```python
from build123d import *

# Parameters (mm, degrees)
F0_W     = 126
F0_H     = 73
F1_DEPTH = 2
F2_W     = 1.7
F2_H     = 1.5
F2_W_2   = 19.1
F2_H_2   = 70
F3_DEPTH = 19
F5_DEPTH = 100
F6_R     = 0.1


with BuildPart() as f1:
    # F0 (on Top) → F1 (new body)
    with BuildSketch(Plane.XY):
        Rectangle(F0_W, F0_H)
    extrude(amount=F1_DEPTH)

    # F2 (on face) → F3 (join)
    with BuildSketch(Plane.XY.offset(2)):
        Polygon((42.4, 35), (61.5, 35), (61.5, -35), (42.4, -35), (42.4, -36.5), (63, -36.5), (63, 36.5), (42.4, 36.5), align=None)
        with Locations((41.55, 35.75)):
            Rectangle(F2_W, F2_H)
        with Locations((31.15, 35.75)):
            Rectangle(F2_W_2, F2_H)
        with Locations((41.55, -35.75)):
            Rectangle(F2_W, F2_H)
        with Locations((20.75, 35.75)):
            Rectangle(F2_W, F2_H)
        with Locations((31.15, -35.75)):
            Rectangle(F2_W_2, F2_H)
        with Locations((10.35, 35.75)):
            Rectangle(F2_W_2, F2_H)
        with Locations((20.75, -35.75)):
            Rectangle(F2_W, F2_H)
        with Locations((-0.05, 35.75)):
            Rectangle(F2_W, F2_H)
        with Locations((10.35, -35.75)):
            Rectangle(F2_W_2, F2_H)
        with Locations((-10.45, 35.75)):
            Rectangle(F2_W_2, F2_H)
        with Locations((-0.05, -35.75)):
            Rectangle(F2_W, F2_H)
        with Locations((-20.85, 35.75)):
            Rectangle(F2_W, F2_H)
        with Locations((-10.45, -35.75)):
            Rectangle(F2_W_2, F2_H)
        with Locations((-31.25, 35.75)):
            Rectangle(F2_W_2, F2_H)
        with Locations((-20.85, -35.75)):
            Rectangle(F2_W, F2_H)
        with Locations((-41.65, 35.75)):
            Rectangle(F2_W, F2_H)
        with Locations((-31.25, -35.75)):
            Rectangle(F2_W_2, F2_H)
        Polygon((-61.5, 35), (-42.5, 35), (-42.5, 36.5), (-63, 36.5), (-63, -36.5), (-42.5, -36.5), (-42.5, -35), (-61.5, -35), align=None)
        with Locations((-41.65, -35.75)):
            Rectangle(F2_W, F2_H)
        with Locations((-41.65, 0)):
            Rectangle(F2_W, F2_H_2)
        with Locations((-20.85, 0)):
            Rectangle(F2_W, F2_H_2)
        with Locations((-0.05, 0)):
            Rectangle(F2_W, F2_H_2)
        with Locations((20.75, 0)):
            Rectangle(F2_W, F2_H_2)
        with Locations((41.55, 0)):
            Rectangle(F2_W, F2_H_2)
    extrude(amount=F3_DEPTH)

    # F4 (on face) → F5 (cut)
    with BuildSketch(Plane.XZ.offset(36.5)):
        with BuildLine():
            ThreePointArc((-49.5, 10.5), (-52, 13), (-54.5, 10.5))
            Line((-54.5, 10.5), (-49.5, 10.5))
        make_face()
        with BuildLine():
            ThreePointArc((54.5, 10.5), (52, 13), (49.5, 10.5))
            Line((49.5, 10.5), (54.5, 10.5))
        make_face()
        with BuildLine():
            Line((54.5, 10.5), (49.5, 10.5))
            ThreePointArc((49.5, 10.5), (52, 8), (54.5, 10.5))
        make_face()
        with BuildLine():
            ThreePointArc((33.8, 10.5), (31.3, 13), (28.8, 10.5))
            Line((28.8, 10.5), (33.8, 10.5))
        make_face()
        with BuildLine():
            Line((33.8, 10.5), (28.8, 10.5))
            ThreePointArc((28.8, 10.5), (31.3, 8), (33.8, 10.5))
        make_face()
        with BuildLine():
            ThreePointArc((13.1, 10.5), (10.6, 13), (8.1, 10.5))
            Line((8.1, 10.5), (13.1, 10.5))
        make_face()
        with BuildLine():
            Line((13.1, 10.5), (8.1, 10.5))
            ThreePointArc((8.1, 10.5), (10.6, 8), (13.1, 10.5))
        make_face()
        with BuildLine():
            ThreePointArc((-8.1, 10.5), (-10.6, 13), (-13.1, 10.5))
            Line((-13.1, 10.5), (-8.1, 10.5))
        make_face()
        with BuildLine():
            Line((-8.1, 10.5), (-13.1, 10.5))
            ThreePointArc((-13.1, 10.5), (-10.6, 8), (-8.1, 10.5))
        make_face()
        with BuildLine():
            ThreePointArc((-28.8, 10.5), (-31.3, 13), (-33.8, 10.5))
            Line((-33.8, 10.5), (-28.8, 10.5))
        make_face()
        with BuildLine():
            Line((-28.8, 10.5), (-33.8, 10.5))
            ThreePointArc((-33.8, 10.5), (-31.3, 8), (-28.8, 10.5))
        make_face()
        with BuildLine():
            Line((-49.5, 10.5), (-54.5, 10.5))
            ThreePointArc((-54.5, 10.5), (-52, 8), (-49.5, 10.5))
        make_face()
    extrude(amount=-F5_DEPTH, mode=Mode.SUBTRACT)

    # F6
    f6_edges = [f1.edges().sort_by_distance(p)[0] for p in [
        (-63, -36.5, 10.5),
        (63, -36.5, 10.5),
        (63, 36.5, 10.5),
        (-63, 36.5, 10.5),
    ]]
    fillet(f6_edges, radius=F6_R)


solid = f1.part
```
Verification items for the finished model (mm, model axes). A direction names the side the tool comes from. Give positions to 0.01 mm unless a question says otherwise; leave off trailing zeros. Order: outer loops, then holes, each group sorted by start corner. A loop starts at its lowest first (then second) coordinate and runs counter-clockwise, first axis right, second up. Notation, with made-up numbers: M 69.25,-39 L 104.25,-39 A5 cw 104.25,-33 Z; hole C 25,-11.5 d7. An arc over 180 degrees is marked long. Return JSON: item names as keys, results as strings. Group by question number.
1) Scan lines: line 1 (Y direction, x = -13, z = 6.5); line 2 (Z direction, x = 52, y = 36); line 3 (Z direction, x = 3, y = 7). Record each from-to range of solid material in increasing order.
2) Mould release check, pull along Y, two halves, no side actions. Record for faces 1 (the face through (-11, 0, 2)), 2 (the face through (63, -1, 10)), 3 (the face through (-1, -36.5, 10)): pulls with the +Y half, pulls with the -Y half, needs draft (parallel to the pull), parting line crosses it, or undercut.
3) Access from +Z, -Z, +X, -X, +Y, -Y to the whole of each face (thin tool, end or side, straight path). Record for faces 4 (the face through (0, 11, 21)), 5 (the face through (-51.9, -35, 13.5)).
4) Go/stop test with flat-tipped pins: pin 1 Ø4 at (x, z) = (-10.6, 10.5) entering from +Y; pin 2 Ø9.5 at (x, y) = (-12.5, 0) entering from +Z. Record where each tip stops, or that it passes through.
5) Section check C-C on x = -25. Record the cut outline in (y, z).
6) Section check A-A on x = 31.3. Record the cut outline in (y, z), and give its area (3 significant figures).
7) Section check B-B on z = 18.5. Give the number of separate pieces and of enclosed holes in the cut face, and give its area (3 significant figures).
8) Section check D-D on y = -16. Record the cut outline in (x, z).
Answer block:
{
 "1": {"line 1": "y = -36.5 to -35, 35 to 36.5", "line 2": "z = 0 to 8, 13 to 21", "line 3": "z = 0 to 2"},
 "2": {"face 1": "undercut", "face 2": "needs draft", "face 3": "pulls with the -Y half"},
 "3": {"face 4": "+Z, +X, -X, +Y, -Y", "face 5": "+Z"},
 "4": {"pin 1": "passes through", "pin 2": "stops at z = 2"},
 "5": {"outline": "M -36.5,0 L 36.5,0 L 36.5,21 L 35,21 L 35,2 L -35,2 L -35,21 L -36.5,21 Z"},
 "6": {"outline": "M -36.5,0 L 36.5,0 L 36.5,8 L 35,8 L 35,2 L -35,2 L -35,8 L -36.5,8 Z; M -36.5,13 L -35,13 L -35,21 L -36.5,21 Z; M 35,13 L 36.5,13 L 36.5,21 L 35,21 Z", "area": "188 mm^2"},
 "7": {"separate pieces": "1", "enclosed holes": "6", "area": "1,180 mm^2"},
 "8": {"outline": "M -63,0 L 63,0 L 63,21 L 61.5,21 L 61.5,2 L 42.4,2 L 42.4,21 L 40.7,21 L 40.7,2 L 21.6,2 L 21.6,21 L 19.9,21 L 19.9,2 L 0.8,2 L 0.8,21 L -0.9,21 L -0.9,2 L -20,2 L -20,21 L -21.7,21 L -21.7,2 L -40.8,2 L -40.8,21 L -42.5,21 L -42.5,2 L -61.5,2 L -61.5,21 L -63,21 Z"}
}
